from build123d import *

# Parameters (mm, degrees)
SKIZZE1_R                       = 2.7
AUFSATZ_LINEAR_AUSTRAGEN1_DEPTH = 2.95
SKIZZE2_R                       = 1.45
AUFSATZ_LINEAR_AUSTRAGEN2_DEPTH = 12
FASE1_SIZE                      = 0.3
SCHNITT_LINEAR_AUSTRAGEN1_DEPTH = 2.5


with BuildPart() as part:
    # Skizze1 → Aufsatz-Linear austragen1 (new body)
    with BuildSketch(Plane.XY):
        Circle(SKIZZE1_R)
    extrude(amount=AUFSATZ_LINEAR_AUSTRAGEN1_DEPTH)

    # Skizze2 → Aufsatz-Linear austragen2 (add)
    with BuildSketch(Plane.XY.offset(2.95)):
        Circle(SKIZZE2_R)
    extrude(amount=AUFSATZ_LINEAR_AUSTRAGEN2_DEPTH)

    # Fase1
    fase1_edges = [part.edges().sort_by_distance(p)[0] for p in [
        (-2.7, 0, 0),
        (-2.7, 0, 2.95),
        (-1.45, 0, 14.95),
    ]]
    chamfer(fase1_edges, length=FASE1_SIZE)

    # Skizze3 → Schnitt-Linear austragen1 (cut)
    with BuildSketch(Plane(origin=(0, 0, 0), x_dir=(-1, 0, 0), z_dir=(0, 0, -1))):
        Polygon((1.25, 0.721687836), (0, 1.443375673), (-1.25, 0.721687836), (-1.25, -0.721687836), (0, -1.443375673), (1.25, -0.721687836), align=None)
    extrude(amount=-SCHNITT_LINEAR_AUSTRAGEN1_DEPTH, mode=Mode.SUBTRACT)


solid = part.part
Verification items for the finished model (mm, model axes). A direction names the side the tool comes from. Round coordinates to 2 decimals unless told otherwise and drop trailing zeros. Loops run counter-clockwise (first coordinate to the right, second up) from the corner with the lowest first, then second, coordinate; pieces in that order, holes last. Notation, with made-up numbers: (66, 84) - (88, 84) arc R15 cw to (88, 96) - close; hole circle Ø1 at (-38.75, 84.25). An arc over 180 degrees is marked (long way). Write item = value, one per line.
Q1. Depth check by flat-ended pin: pin 1 (3 mm diameter, centred on y = 0.5, z = 10, fed in from +X); pin 2 (0.8 mm diameter, centred on x = -0.5, y = -0.5, fed in from -Z); pin 3 (2 mm diameter, centred on y = -0.5, z = 9.5, fed in from -X). Enter the tip coordinate at first touch or a pass-through.
Here are the results:
pin_1 = 1.45
pin_2 = 2.5
pin_3 = -1.45
Q2. Material ranges on L1, parallel to X at y = -0.15, z = 12.5; L2, parallel to Z at x = -1.75, y = -0.35; L3, parallel to Z at x = -0.3, y = 0.1, recorded low to high.
Here are the results:
L1 = -1.44 to 1.44
L2 = 0 to 2.95
L3 = 2.5 to 14.95
Q3. Sectioned sample at B-B on z = 3.25. Record the boundary of the cut face in (x, y), plus the area to 3 significant figures.
Here are the results:
outline = circle Ø2.9 at (0, 0)
area = 6.61 mm^2
Q4. Sectioned sample at A-A on y = 0. Record the boundary of the cut face in (x, z).
Here are the results:
outline = (-2.7, 0.3) - (-2.4, 0) - (-1.25, 0) - (-1.25, 2.5) - (1.25, 2.5) - (1.25, 0) - (2.4, 0) - (2.7, 0.3) - (2.7, 2.65) - (2.4, 2.95) - (1.45, 2.95) - (1.45, 14.65) - (1.15, 14.95) - (-1.15, 14.95) - (-1.45, 14.65) - (-1.45, 2.95) - (-2.4, 2.95) - (-2.7, 2.65) - close
Q5. Mould release check, pull along Y, two halves, no side actions. Record for faces 1 (the flat face through (0, -2, 2.95)), 2 (the flat face through (-0.616, -1.088, 1.232)), 3 (the cylindrical face through (-1.45, 0.06, 8.72)): +Y half, -Y half, draft (parallel to the pull), parting line (faces both ways), or undercut.
Here are the results:
face_1 = draft
face_2 = undercut
face_3 = parting line
Q6. Tool access check on faces 4 (the flat face through (-1.25, 0, 1)), 5 (the cylindrical face through (-0.585, -2.636, 1.459)). Record the directions out of +Z, -Z, +X, -X, +Y, -Y that give a thin tool (end or side, any length) a straight path to the whole face; none if there is none.
Here are the results:
face_4 = -Z
face_5 = +Z, -Z
